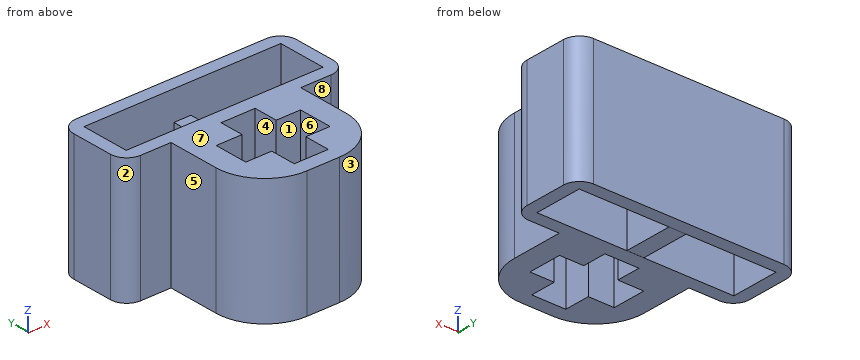
from build123d import *

# Parameters (mm, degrees)
SKETCH1_W           = 8
SKETCH1_H           = 7
BOSS_EXTRUDE1_DEPTH = 7.76
CUT_EXTRUDE3_DEPTH  = 8.76
SKETCH7_W           = 7.76
SKETCH7_H           = 0.8
BOSS_EXTRUDE2_DEPTH = 2.87
SKETCH9_W           = 7.76
SKETCH9_H           = 0.8
BOSS_EXTRUDE3_DEPTH = 2.87
SKETCH10_W          = 0.8
SKETCH10_H          = 7.76
BOSS_EXTRUDE4_DEPTH = 3
SKETCH11_W          = 0.8
SKETCH11_H          = 7.76
BOSS_EXTRUDE5_DEPTH = 3
SKETCH12_W          = 13.74
SKETCH12_H          = 7.76
BOSS_EXTRUDE6_DEPTH = 0.8
BOSS_EXTRUDE7_REACH = 5.8
FILLET4_R           = 1
FILLET5_R           = 1
FILLET6_R           = 1
FILLET7_R           = 1
FILLET8_R           = 3
FILLET9_R           = 3


with BuildPart() as part:
    # Sketch1 → Boss-Extrude1 (new body)
    with BuildSketch(Plane.XY):
        Rectangle(SKETCH1_W, SKETCH1_H)
    extrude(amount=BOSS_EXTRUDE1_DEPTH)

    # Sketch6 → Cut-Extrude3 (cut, through all)
    with BuildSketch(Plane.XY.offset(7.76)):
        Polygon((1.1, -1), (2.6, -1), (2.6, 1.1), (1.1, 1.1), (1.1, 2.6), (-1, 2.6), (-1, 1.1), (-2.6, 1.1), (-2.6, -1), (-1, -1), (-1, -2.6), (1.1, -2.6), align=None)
    extrude(amount=-CUT_EXTRUDE3_DEPTH, mode=Mode.SUBTRACT)

    # Sketch7 → Boss-Extrude2 (add)
    with BuildSketch(Plane.ZY.offset(4)):
        with Locations((3.88, 3.1)):
            Rectangle(SKETCH7_W, SKETCH7_H)
    extrude(amount=BOSS_EXTRUDE2_DEPTH)

    # Sketch9 → Boss-Extrude3 (add)
    with BuildSketch(Plane(origin=(4, 0, 0), x_dir=(0, 0, -1), z_dir=(1, 0, 0))):
        with Locations((-3.88, 3.1)):
            Rectangle(SKETCH9_W, SKETCH9_H)
    extrude(amount=BOSS_EXTRUDE3_DEPTH)

    # Sketch10 → Boss-Extrude4 (add)
    with BuildSketch(Plane(origin=(0, 3.5, 0), x_dir=(1, 0, 0), z_dir=(0, 1, 0))):
        with Locations((6.47, -3.88)):
            Rectangle(SKETCH10_W, SKETCH10_H)
    extrude(amount=BOSS_EXTRUDE4_DEPTH)

    # Sketch11 → Boss-Extrude5 (add)
    with BuildSketch(Plane(origin=(0, 3.5, 0), x_dir=(1, 0, 0), z_dir=(0, 1, 0))):
        with Locations((-6.47, -3.88)):
            Rectangle(SKETCH11_W, SKETCH11_H)
    extrude(amount=BOSS_EXTRUDE5_DEPTH)

    # Sketch12 → Boss-Extrude6 (add)
    with BuildSketch(Plane(origin=(0, 6.5, 0), x_dir=(1, 0, 0), z_dir=(0, 1, 0))):
        with Locations((0, -3.88)):
            Rectangle(SKETCH12_W, SKETCH12_H)
    extrude(amount=BOSS_EXTRUDE6_DEPTH)

    # Sketch14 → Boss-Extrude7 (add, up to next)
    with BuildSketch(Plane(origin=(0, 3.5, 0), x_dir=(1, 0, 0), z_dir=(0, 1, 0)), mode=Mode.PRIVATE) as boss_extrude7_sk1:
        Polygon((0.525000003, -0.003794521), (-0.524999997, -0.003794521), (-0.524994746, -5.96), (0.525005254, -5.96), align=None)
    boss_extrude7_tool1 = extrude(boss_extrude7_sk1.sketch, amount=BOSS_EXTRUDE7_REACH, mode=Mode.PRIVATE) - part.part
    add(boss_extrude7_tool1.solids().sort_by_distance((3e-06, 3.5, 2.981897))[0])

    # Fillet4
    fillet4_edges = [part.edges().sort_by_distance(p)[0] for p in [
        (-6.87, 7.3, 3.88),
    ]]
    fillet(fillet4_edges, radius=FILLET4_R)

    # Fillet5
    fillet5_edges = [part.edges().sort_by_distance(p)[0] for p in [
        (6.87, 7.3, 3.88),
    ]]
    fillet(fillet5_edges, radius=FILLET5_R)

    # Fillet6
    fillet6_edges = [part.edges().sort_by_distance(p)[0] for p in [
        (-6.87, 2.7, 3.88),
    ]]
    fillet(fillet6_edges, radius=FILLET6_R)

    # Fillet7
    fillet7_edges = [part.edges().sort_by_distance(p)[0] for p in [
        (6.87, 2.7, 3.88),
    ]]
    fillet(fillet7_edges, radius=FILLET7_R)

    # Fillet8
    fillet8_edges = [part.edges().sort_by_distance(p)[0] for p in [
        (4, -3.5, 3.88),
    ]]
    fillet(fillet8_edges, radius=FILLET8_R)

    # Fillet9
    fillet9_edges = [part.edges().sort_by_distance(p)[0] for p in [
        (-4, -3.5, 3.88),
    ]]
    fillet(fillet9_edges, radius=FILLET9_R)


solid = part.part
Here's how the part is built. I have some questions about the finished solid (model axes, mm). Face numbers are marked on the shaded views. A direction names the side the tool comes from. Round coordinates to 2 decimals unless told otherwise and drop trailing zeros. Write each loop counter-clockwise with the first axis right and the second up, starting at its lowest first coordinate (ties: lowest second). Pieces come first, ordered by that corner, then holes.
1. Suppose I cut it at C-C (z = 1.75). State how many separate pieces and enclosed holes the cut face has, and give its area (3 significant figures).
2. For the marked faces 5, 6, 7 and 8, which set-ups out of +Z, -Z, +X, -X, +Y, -Y let a thin tool reach every point of the face, with its end or its side?
3. Suppose I cut it at D-D (y = 5.5). List the corners of the cut face in (x, z) for me (3 decimals), and give its area (3 significant figures).
4. If we mould it in two halves opening along X, with no side actions, what happens to the marked faces 1, 2, 3 and 4? For each: released by +X, released by -X, zero draft, split by the parting line, or undercut.
5. I need wall thicknesses on L1, parallel to X at y = 3.75, z = 3 (3 decimals); L2, parallel to Y at x = 0, z = 6.25; L3, parallel to Y at x = -5.5, z = 4. Which ranges of each line are inside material? Lowest first, please.
6. Suppose I cut it at A-A (y = 2). List the corners of the cut face in (x, z) for me.
7. Will these pins go through, and if not, where does the flat tip stop? pin 1 Ø0.5 at (x, y) = (0, 5.5) entering from +Z; pin 2 Ø4 at (y, z) = (1, 6) entering from +X; pin 3 Ø0.6 at (y, z) = (0, 4.5) entering from -X.
8. Suppose I cut it at B-B (x = 4.25). List the corners of the cut face in (y, z) for me.
Answer sheet:
1. separate pieces: 1
1. enclosed holes: 3
1. area: 57.4 mm2
2. face 5: +Z, -Z, -X, -Y
2. face 6: +Z, -Z
2. face 7: +Z, +X, -X, +Y, -Y
2. face 8: +Z, -Z, +X, -Y
3. outline: (-6.87, 0) - (-6.07, 0) - (-6.07, 7.76) - (-6.87, 7.76) - close; (-0.525, 0.004) - (0.525, 0.004) - (0.525, 5.96) - (-0.525, 5.96) - close; (6.07, 0) - (6.87, 0) - (6.87, 7.76) - (6.07, 7.76) - close
3. area: 18.7 mm2
4. face 1: undercut
4. face 2: released by -X
4. face 3: released by +X
4. face 4: undercut
5. L1: x = -6.87 to -6.07, -0.525 to 0.525, 6.07 to 6.87
5. L2: y = -3.5 to -2.6, 2.6 to 3.5, 6.5 to 7.3
5. L3: y = 2.7 to 3.5, 6.5 to 7.3
6. outline: (-4, 0) - (-1, 0) - (-1, 7.76) - (-4, 7.76) - close; (1.1, 0) - (4, 0) - (4, 7.76) - (1.1, 7.76) - close
7. pin 1: stops at z = 5.96
7. pin 2: stops at x = 6.58
7. pin 3: stops at x = -4
8. outline: (2.7, 0) - (3.5, 0) - (3.5, 7.76) - (2.7, 7.76) - close; (6.5, 0) - (7.3, 0) - (7.3, 7.76) - (6.5, 7.76) - close
